from build123d import *

# Parameters (mm, degrees)
SKETCH1_R           = 6.15
SKETCH1_R_2         = 1.65
BOSS_EXTRUDE1_DEPTH = 60
CUT_EXTRUDE1_DEPTH  = 57
SKETCH3_R           = 1.5
CUT_EXTRUDE2_DEPTH  = 81.597766718


with BuildPart() as part:
    # Sketch1 → Boss-Extrude1 (new body)
    with BuildSketch(Plane.XY):
        with BuildLine():
            Line((-21, 0), (-21, -19))
            Line((-21, -19), (-36, -19))
            Line((-36, -19), (-36, -22))
            Line((-36, -22), (36, -22))
            Line((36, -22), (36, -19))
            Line((36, -19), (21, -19))
            Line((21, -19), (21, 0))
            ThreePointArc((21, 0), (0, 21), (-21, 0))
        make_face()
        with Locations((0, -7)):
            Circle(SKETCH1_R, mode=Mode.SUBTRACT)
        with Locations((-15.5, 0)):
            Circle(SKETCH1_R_2, mode=Mode.SUBTRACT)
        with Locations((-7.75, 13.423393759)):
            Circle(SKETCH1_R_2, mode=Mode.SUBTRACT)
        with Locations((7.75, 13.423393759)):
            Circle(SKETCH1_R_2, mode=Mode.SUBTRACT)
        with Locations((15.5, 0)):
            Circle(SKETCH1_R_2, mode=Mode.SUBTRACT)
        with Locations((7.75, -13.423393759)):
            Circle(SKETCH1_R_2, mode=Mode.SUBTRACT)
        with Locations((-7.75, -13.423393759)):
            Circle(SKETCH1_R_2, mode=Mode.SUBTRACT)
    extrude(amount=BOSS_EXTRUDE1_DEPTH)

    # Sketch2 → Cut-Extrude1 (cut)
    with BuildSketch(Plane.XY.offset(60)):
        with BuildLine():
            Line((-18.5, 0), (-18.5, -19))
            Line((-18.5, -19), (18.5, -19))
            Line((18.5, -19), (18.5, 0))
            ThreePointArc((18.5, 0), (0, 18.5), (-18.5, 0))
        make_face()
    extrude(amount=-CUT_EXTRUDE1_DEPTH, mode=Mode.SUBTRACT)

    # Sketch3 → Cut-Extrude2 (cut, through all)
    with BuildSketch(Plane(origin=(0, -19, 0), x_dir=(1, 0, 0), z_dir=(0, 1, 0))):
        with Locations(Location((-28.5, -30, 0), (0, 0, 270))):
            Circle(SKETCH3_R)
        with Locations(Location((-28.5, -6, 0), (0, 0, 270))):
            Circle(SKETCH3_R)
        with Locations(Location((-28.5, -54, 0), (0, 0, 270))):
            Circle(SKETCH3_R)
        with Locations(Location((28.5, -54, 0), (0, 0, 90))):
            Circle(SKETCH3_R)
        with Locations(Location((28.5, -6, 0), (0, 0, 90))):
            Circle(SKETCH3_R)
        with Locations(Location((28.5, -30, 0), (0, 0, 90))):
            Circle(SKETCH3_R)
    extrude(amount=-CUT_EXTRUDE2_DEPTH, mode=Mode.SUBTRACT)


solid = part.part
Geometry: final body of the model. Coordinates: model frame, mm. A direction names the side the tool comes from. Round coordinates to 2 decimals unless told otherwise and drop trailing zeros. Loops run counter-clockwise (first coordinate to the right, second up) from the corner with the lowest first, then second, coordinate; pieces in that order, holes last. Notation, with made-up numbers: (-12, -31) -> (7, -31) arc R15 ccw to (7, -7) -> close; hole circle Ø6 at (66.5, 74). An arc over 180 degrees is marked (long way). One line per question, with ' | ' between items. Start each with the question number.
1. Set-up query: faces 1 (the face through (18.5, -10, 32)), 2 (the face through (30.3, -19, 29.6)), 3 (the face through (27.49, -20.48, 31.11)), 4 (the face through (-21, -9, 30)). Return all of +Z, -Z, +X, -X, +Y, -Y with unobstructed straight access to the full face (end or side cutting, diameter ignored); none if empty.
2. Section C-C on z = 33.5. Output: boundary loops of the cut face in (x, y), and give its area (3 significant figures).
3. Section B-B on x = 0. Output: boundary loops of the cut face in (y, z).
4. Section D-D on x = -28.5. Output: boundary loops of the cut face in (y, z), and give its area (3 significant figures).
5. Line query: line 1 along Z through (x, y) = (28.5, -19.75); line 2 along X through (y, z) = (-21, 30); line 3 along X through (y, z) = (-0.5, 11.5). Output: solid intervals per line, ascending. Write a range as [from, to].
6. Mould query, pull axis X, two halves, no side actions, for faces 5 (the face through (0.407, 18.496, 31.899)), 6 (the face through (21, -10, 30)), 7 (the face through (-1, 0, 0)). Classes: pulls with the +X half, pulls with the -X half, needs draft (parallel to the pull), parting line crosses it, or undercut.
7. Section A-A on z = 54. Output: boundary loops of the cut face in (x, y).
8. Contact query for flat-ended pins moving along their axis: pin 1 (1 mm diameter, centred on x = 15.5, z = 36.5, fed in from +Y); pin 2 (4.5 mm diameter, centred on x = -27.5, z = 26, fed in from +Y); pin 3 (5 mm diameter, centred on x = -4.5, y = 4, fed in from +Z); pin 4 (3 mm diameter, centred on x = 5, y = -4, fed in from -Z). Output: stop coordinate, or through.
Returned:
1) face 1: +Z | face 2: +Z, -Z, +X, +Y | face 3: +Y, -Y | face 4: +Z, -Z, -X, +Y
2) outline: (-36, -22) -> (36, -22) -> (36, -19) -> (21, -19) -> (21, 0) arc R21 ccw to (-21, 0) -> (-21, -19) -> (-36, -19) -> close; hole (-18.5, -19) -> (18.5, -19) -> (18.5, 0) arc R18.5 ccw to (-18.5, 0) -> close | area: 466 mm2
3) outline: (-22, 0) -> (-13.15, 0) -> (-13.15, 3) -> (-19, 3) -> (-19, 60) -> (-22, 60) -> close; (-0.85, 0) -> (21, 0) -> (21, 60) -> (18.5, 60) -> (18.5, 3) -> (-0.85, 3) -> close
4) outline: (-22, 0) -> (-19, 0) -> (-19, 4.5) -> (-22, 4.5) -> close; (-22, 7.5) -> (-19, 7.5) -> (-19, 28.5) -> (-22, 28.5) -> close; (-22, 31.5) -> (-19, 31.5) -> (-19, 52.5) -> (-22, 52.5) -> close; (-22, 55.5) -> (-19, 55.5) -> (-19, 60) -> (-22, 60) -> close | area: 153 mm2
5) line 1: z = [0, 4.5], [7.5, 28.5], [31.5, 52.5], [55.5, 60] | line 2: x = [-36, -30], [-27, 27], [30, 36] | line 3: x = [-21, -18.5], [18.5, 21]
6) face 5: undercut | face 6: pulls with the +X half | face 7: needs draft
7) outline: (-36, -22) -> (-30, -22) -> (-30, -19) -> (-36, -19) -> close; (-27, -22) -> (27, -22) -> (27, -19) -> (21, -19) -> (21, 0) arc R21 ccw to (-21, 0) -> (-21, -19) -> (-27, -19) -> close; (30, -22) -> (36, -22) -> (36, -19) -> (30, -19) -> close; hole (-18.5, -19) -> (18.5, -19) -> (18.5, 0) arc R18.5 ccw to (-18.5, 0) -> close
8) pin 1: stops at y = 14.7 | pin 2: stops at y = -19 | pin 3: stops at z = 3 | pin 4: stops at z = 0
